Autodesk Inventor part; units mm, degrees
ref_plane "YZ Plane" through (0, 0, 0) normal (1, 0, 0) x (0, 1, 0)
ref_plane "XZ Plane" through (0, 0, 0) normal (0, 1, 0) x (-1, 0, 0)
ref_plane "XY Plane" through (0, 0, 0) normal (0, 0, 1) x (1, 0, 0)
sketch "Sketch1" plane through (0, 0, 0) normal (0, 1, 0) x (-1, 0, 0)
  line L0 (0, 25) -> (25, 25)
  line L1 (25, 25) -> (25, 0)
  line L2 (25, 25) -> (23, 25)
  line L3 (25, 23) -> (25, 25)
  circle A0 centre (23, 23) radius 1.5
  circle A1 centre (18.0503, 18.0503) radius 1.5
  line L4 (0, 25) -> (0, 8.5)
  line L5 (8.5, 0) -> (25, 0)
  arc A2 (8.5, 0) -> (0, 8.5) centre (0, 0) ccw
  dimension "d5" = 3
  dimension "d7" = 3
extrude "Extrusion1" add sketch "Sketch1" along normal blind 1
pattern_circular "Circular Pattern1" count 4 over 360 about axis through (0, 0, 0) along (0, 1, 0) of "Extrusion1"
fillet "Fillet1" radius 2 4 edges at (-25, 0.5, 25) (-25, 0.5, -25) (25, 0.5, 25) (25, 0.5, -25)
properties part number "POWER_distribution"
Model file for the job. Use its own axes, mm. Round coordinates to 2 decimals unless told otherwise and drop trailing zeros. Loops run counter-clockwise (first coordinate to the right, second up) from the corner with the lowest first, then second, coordinate; pieces in that order, holes last. Notation, with made-up numbers: (-31.5, 12) -> (-17.5, 12) arc R20 cw to (-17.5, 40) -> close; hole circle Ø2 at (-21, 43.25). An arc over 180 degrees is marked (long way). Answer as CSV lines item,"result". Start each with the question number.
1) Mould opens along X. For faces 1 (the face through (21.99, 0.49, 21.89)), 2 (the face through (-24.4, 0.51, -24.43)), 3 (the face through (0, 1, -11)) say: +X half, -X half, draft (parallel to the pull), parting line (faces both ways), or undercut.
2) Probe line 1 along X through (y, z) = (0.1, 18); line 2 along Z through (x, y) = (-18.5, 0.1); line 3 along Z through (x, y) = (-17, 0.65). List the from-to ranges inside material, lowest first.
3) Slice it at B-B (z = 0). List the corners of the cut face in (x, y).
4) Slice it at C-C (y = 0.55). State how many separate pieces and enclosed holes the cut face has, plus the area to 3 significant figures.
5) Slice it at A-A (x = -4). List the corners of the cut face in (y, z).
Filled in:
1,face 1,"undercut"
1,face 2,"-X half"
1,face 3,"draft"
2,line 1,"x = -25 to -19.55, -16.55 to 16.55, 19.55 to 25"
2,line 2,"z = -25 to -19.48, -16.62 to 16.62, 19.48 to 25"
2,line 3,"z = -25 to -19.12, -16.98 to 16.98, 19.12 to 25"
3,outline,"(-25, 0) -> (-8.5, 0) -> (-8.5, 1) -> (-25, 1) -> close; (8.5, 0) -> (25, 0) -> (25, 1) -> (8.5, 1) -> close"
4,separate pieces,"1"
4,enclosed holes,"9"
4,area,"2,210 mm2"
5,outline,"(0, -25) -> (1, -25) -> (1, -7.5) -> (0, -7.5) -> close; (0, 7.5) -> (1, 7.5) -> (1, 25) -> (0, 25) -> close"
